Design review of the part built by this model. Coordinates are the model's own, in mm. Give positions to 0.01 mm unless a question says otherwise; leave off trailing zeros. Write each loop counter-clockwise with the first axis right and the second up, starting at its lowest first coordinate (ties: lowest second). Pieces come first, ordered by that corner, then holes.
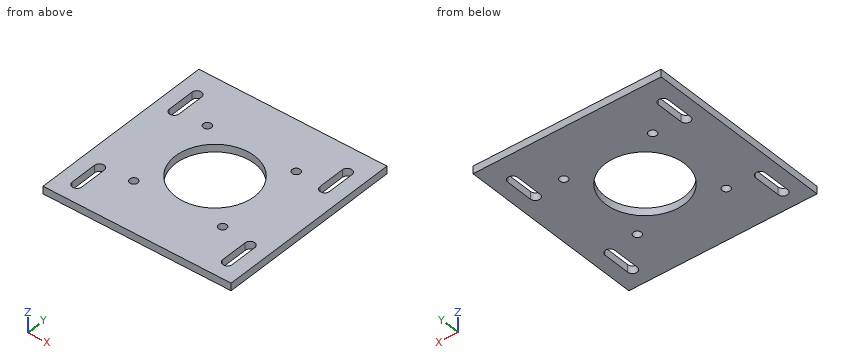
```python
from build123d import *

# Parameters (mm, degrees)
SKETCH1_R           = 2.15
SKETCH1_R_2         = 21
BOSS_EXTRUDE1_DEPTH = 4


with BuildPart() as part:
    # Sketch1 → Boss-Extrude1 (new body)
    with BuildSketch(Plane.XY):
        Polygon((0, 0), (0, 90), (100, 90), (100, 2.372295937), (100, -10), (0, -10), align=None)
        with Locations((26.4, 63.6)):
            Circle(SKETCH1_R, mode=Mode.SUBTRACT)
        with Locations((73.6, 63.6)):
            Circle(SKETCH1_R, mode=Mode.SUBTRACT)
        with Locations((73.6, 16.4)):
            Circle(SKETCH1_R, mode=Mode.SUBTRACT)
        with Locations((26.4, 16.4)):
            Circle(SKETCH1_R, mode=Mode.SUBTRACT)
        with Locations((50, 40)):
            Circle(SKETCH1_R_2, mode=Mode.SUBTRACT)
        with BuildLine():
            Line((7.45, 14.17243776), (7.45, -0.25030049))
            ThreePointArc((7.45, -0.25030049), (10, -2.80030049), (12.55, -0.25030049))
            Line((12.55, -0.25030049), (12.55, 14.17243776))
            ThreePointArc((12.55, 14.17243776), (10, 16.72243776), (7.45, 14.17243776))
        make_face(mode=Mode.SUBTRACT)
        with BuildLine():
            Line((87.45, 62.150571419), (87.45, 76.57330967))
            ThreePointArc((87.45, 76.57330967), (90, 79.12330967), (92.55, 76.57330967))
            Line((92.55, 76.57330967), (92.55, 62.150571419))
            ThreePointArc((92.55, 62.150571419), (90, 59.600571419), (87.45, 62.150571419))
        make_face(mode=Mode.SUBTRACT)
        with BuildLine():
            Line((92.55, 14.17243776), (92.55, -0.25030049))
            ThreePointArc((92.55, -0.25030049), (90, -2.80030049), (87.45, -0.25030049))
            Line((87.45, -0.25030049), (87.45, 14.17243776))
            ThreePointArc((87.45, 14.17243776), (90, 16.72243776), (92.55, 14.17243776))
        make_face(mode=Mode.SUBTRACT)
        with BuildLine():
            Line((12.55, 62.150571419), (12.55, 76.57330967))
            ThreePointArc((12.55, 76.57330967), (10, 79.12330967), (7.45, 76.57330967))
            Line((7.45, 76.57330967), (7.45, 62.150571419))
            ThreePointArc((7.45, 62.150571419), (10, 59.600571419), (12.55, 62.150571419))
        make_face(mode=Mode.SUBTRACT)
    extrude(amount=BOSS_EXTRUDE1_DEPTH)


solid = part.part
```
(1) Clearance check with a flat-ended pin moving along its axis: P1, Ø1.2, axis at y = 72, z = 2.5, coming from the -X side. State where the tip first meets the part, or that it passes through.
Resolved:
P1: stops at x = 0
(2) Consider section A-A, the plane y = 72. Give the boundary of the cut face in (x, z).
Resolved:
outline: (0, 0) - (7.45, 0) - (7.45, 4) - (0, 4) - close; (12.55, 0) - (87.45, 0) - (87.45, 4) - (12.55, 4) - close; (92.55, 0) - (100, 0) - (100, 4) - (92.55, 4) - close
(3) To check wall thickness, follow L1, parallel to Y at x = 73.6, z = 2.65; L2, parallel to X at y = 13, z = 1.45; L3, parallel to X at y = -1, z = 2.1. State the ranges of each line that lie inside material, in increasing order.
Resolved:
L1: y = -10 to 14.25, 18.55 to 61.45, 65.75 to 90
L2: x = 0 to 7.45, 12.55 to 87.45, 92.55 to 100
L3: x = 0 to 7.56, 12.44 to 87.56, 92.44 to 100
(4) Consider section B-B, the plane x = 73.6. Give the boundary of the cut face in (y, z), then the cut area to 3 significant figures.
Resolved:
outline: (-10, 0) - (14.25, 0) - (14.25, 4) - (-10, 4) - close; (18.55, 0) - (61.45, 0) - (61.45, 4) - (18.55, 4) - close; (65.75, 0) - (90, 0) - (90, 4) - (65.75, 4) - close
area: 366 mm2
(5) Consider section C-C, the plane x = 50. Give the boundary of the cut face in (y, z), then the cut area to 3 significant figures.
Resolved:
outline: (-10, 0) - (19, 0) - (19, 4) - (-10, 4) - close; (61, 0) - (90, 0) - (90, 4) - (61, 4) - close
area: 232 mm2
(6) Consider section D-D, the plane y = 40. Give the boundary of the cut face in (x, z), then the cut area to 3 significant figures.
Resolved:
outline: (0, 0) - (29, 0) - (29, 4) - (0, 4) - close; (71, 0) - (100, 0) - (100, 4) - (71, 4) - close
area: 232 mm2
